```python
from build123d import *

# Parameters (mm, degrees)
BOSS_EXTRUDE1_DEPTH = 4
BOSS_EXTRUDE1_DRAFT = 1
SHELL1_T            = -0.5
SKETCH2_R           = 2
BOSS_EXTRUDE2_DEPTH = 5.5
BOSS_EXTRUDE2_TAPER = 1.5
CIRPATTERN1_COUNT   = 4
SKETCH4_R           = 1.605977431
CUT_EXTRUDE1_DEPTH  = 5.5
CUT_EXTRUDE1_DRAFT  = 1.5


with BuildPart() as part:
    # Sketch1 → Boss-Extrude1 (with draft: the straight prism first)
    with BuildSketch(Plane(origin=(0, 0, 0), x_dir=(1, 0, 0), z_dir=(0, 1, 0))):
        with BuildLine():
            Line((-7.5, -6.375), (7.5, -6.375))
            ThreePointArc((7.5, -6.375), (8.207106781, -6.082106781), (8.5, -5.375))
            Line((8.5, -5.375), (8.5, 5.375))
            ThreePointArc((8.5, 5.375), (8.207106781, 6.082106781), (7.5, 6.375))
            Line((7.5, 6.375), (-7.5, 6.375))
            ThreePointArc((-7.5, 6.375), (-8.207106781, 6.082106781), (-8.5, 5.375))
            Line((-8.5, 5.375), (-8.5, -5.375))
            ThreePointArc((-8.5, -5.375), (-8.207106781, -6.082106781), (-7.5, -6.375))
        make_face()
    extrude(amount=-BOSS_EXTRUDE1_DEPTH)
    # Boss-Extrude1: the draft: its side faces are tilted about the plane it starts from
    boss_extrude1_sides = [part.faces().sort_by_distance(p)[0] for p in [
        (0, -2, 6.375),
        (8.207106781, -2, 6.082106781),
        (8.5, -2, 0),
        (8.207106781, -2, -6.082106781),
        (0, -2, -6.375),
        (-8.207106781, -2, -6.082106781),
        (-8.5, -2, 0),
        (-8.207106781, -2, 6.082106781),
    ]]
    draft(boss_extrude1_sides, Plane(origin=(0, 0, 0), x_dir=(1, 0, 0), z_dir=(0, 1, 0)), BOSS_EXTRUDE1_DRAFT)

    # Shell1
    shell1_openings = [part.faces().sort_by_distance(p)[0] for p in [
        (0, -4, 0),
    ]]
    offset(amount=SHELL1_T, openings=shell1_openings, kind=Kind.INTERSECTION)

    # Sketch2 → Boss-Extrude2 (add)
    with BuildSketch(Plane.XZ.offset(0.5)):
        Circle(SKETCH2_R)
    extrude(amount=BOSS_EXTRUDE2_DEPTH, taper=BOSS_EXTRUDE2_TAPER)

    # Rib1: read off the stored shape, not the designer's step
    # Rib1: loft between two sections, ruled curve by curve
    rib1_from = [
        Edge.make_line((1.98200897, -0.5, 0.267657325), (3, -0.5, 0.25)),
        Edge.make_line((1.98200897, -0.5, -0.267657325), (3, -0.5, -0.25)),
        Edge.make_line((3, -0.5, -0.25), (3, -0.5, 0.25)),
        Edge.make_line((1.98200897, -0.5, -0.267657325), (1.98200897, -0.5, 0.267657325)),
    ]
    rib1_to = [
        Edge.make_line((1.837759395, -6, 0.259408234), (2.380168761, -6, 0.25)),
        Edge.make_line((1.837759395, -6, -0.259408234), (2.380168761, -6, -0.25)),
        Edge.make_line((2.380168761, -6, -0.25), (2.380168761, -6, 0.25)),
        Edge.make_line((1.837759395, -6, -0.259408234), (1.837759395, -6, 0.259408234)),
    ]
    rib1 = Solid(Shell([*[Face.make_surface_from_curves(rib1_from[k], rib1_to[k]) for k in range(4)], Face(Wire(rib1_from)), Face(Wire(rib1_to))]))
    add(rib1)

    # CirPattern1: Rib1 ×4 about axis
    cirpattern1_axis = Axis((0, 0, 0), (0, 1, 0))
    for i in range(1, CIRPATTERN1_COUNT):
        add(rib1.rotate(cirpattern1_axis, i * 360 / CIRPATTERN1_COUNT))


with BuildPart() as cut_extrude1_tool:
    # Sketch4 → Cut-Extrude1 (with draft: the straight prism first)
    with BuildSketch(Plane.XZ.offset(6)):
        Circle(SKETCH4_R)
    extrude(amount=-CUT_EXTRUDE1_DEPTH)
    # Cut-Extrude1: the draft: its side faces are tilted about the plane it starts from
    cut_extrude1_sides = [cut_extrude1_tool.faces().sort_by_distance(p)[0] for p in [
        (-1.605977431, -3.25, 0),
    ]]
    draft(cut_extrude1_sides, Plane.XZ.offset(6), CUT_EXTRUDE1_DRAFT)


with BuildPart() as part_1:
    add(part.part)

    # Cut-Extrude1: cut by cut_extrude1_tool
    add(cut_extrude1_tool.part, mode=Mode.SUBTRACT)


solid = part_1.part
```
Here's how the part is built. I have some questions about the finished solid (model axes, mm). A direction names the side the tool comes from. Give positions to 0.01 mm unless a question says otherwise; leave off trailing zeros. Loops run counter-clockwise (first coordinate to the right, second up) from the corner with the lowest first, then second, coordinate; pieces in that order, holes last. Notation, with made-up numbers: M 32.25,8 L 37.25,8 A24 ccw 37.25,21 Z; hole C 9,43 d9. An arc over 180 degrees is marked long. Put each result on its own line as item: value. Start each with the question number.
(1) I want a section at B-B on y = -3. State how many separate pieces and enclosed holes the cut face has, then the cut area to 3 significant figures.
(2) Will these pins go through, and if not, where does the flat tip stop? pin 1 Ø1 at (x, z) = (-0.5, -0.5) entering from -Y; pin 2 Ø5 at (x, z) = (-3, 4.5) entering from -Y; pin 3 Ø1.5 at (x, y) = (5, -5) entering from -Z.
(3) I want a section at C-C on x = -5.5. Please give me the cut outline in (y, z) (3 decimals).
(4) I need wall thicknesses on line 1 along X through (y, z) = (-3.5, -0.75); line 2 along Y through (x, z) = (-7.5, 4); line 3 along X through (y, z) = (-3.25, 2.5). Which ranges of each line are inside material? Lowest first, please. Write a range as [from, to].
(5) I want a section at A-A on z = 4.25. Please give me the cut outline in (x, y).
(6) For faces 5 (the conical face through (1.35, -3.288, -1.375)), 6 (the conical face through (-0.218, -3.288, 1.663)), 7 (the flat face through (2, -6, 0)), which set-ups out of +Z, -Z, +X, -X, +Y, -Y let a thin tool reach every point of the face, with its end or its side?
(7) If we mould it in two halves opening along X, with no side actions, what happens to faces 1 (the conical face through (8.24, -1.97, -6.1)), 2 (the conical face through (-8.223, -1.972, -6.114)), 3 (the flat face through (0, -0.5, 0)), 4 (the flat face through (0, -4, -6.2))? For each: +X half, -X half, draft (parallel to the pull), parting line (faces both ways), or undercut.
Answer block:
1. separate pieces: 2
1. enclosed holes: 2
1. area: 32.7 mm^2
2. pin 1: y = -0.5
2. pin 2: y = -4
2. pin 3: through
3. outline: M -4,-6.445 L 0,-6.375 L 0,6.375 L -4,6.445 L -4,5.945 L -0.5,5.884 L -0.5,-5.884 L -4,-5.945 Z
4. line 1: [-8.56, -8.06], [-1.77, -1.49], [1.49, 1.77], [8.06, 8.56]
4. line 2: [-0.5, 0]
4. line 3: [-8.56, -8.06], [-0.25, 0.25], [8.06, 8.56]
5. outline: M -8.57,-4 L -8.07,-4 L -8.01,-0.5 L 8.01,-0.5 L 8.07,-4 L 8.57,-4 L 8.5,0 L -8.5,0 Z
6. face 5: -Y
6. face 6: none
6. face 7: +Z, -Z, +X, -X, -Y
7. face 1: +X half
7. face 2: -X half
7. face 3: undercut
7. face 4: draft
